Design review of the part built by this model. Coordinates are the model's own, in mm. Give positions to 0.01 mm unless a question says otherwise; leave off trailing zeros. Write each loop counter-clockwise with the first axis right and the second up, starting at its lowest first coordinate (ties: lowest second). Pieces come first, ordered by that corner, then holes. Notation, with made-up numbers: (48, 27) -> (62, 27) arc R27 ccw to (62, 56) -> close; hole circle Ø6 at (38.25, 7.25). An arc over 180 degrees is marked (long way). Answer as a JSON object with one key per item and string values.
```python
from build123d import *

# Parameters (mm, degrees)
F0_R     = 69.85
F0_R_2   = 11.1125
F1_DEPTH = 12.7
F2_SIZE  = 1.5875
F3_SIZE  = 1.5875


with BuildPart() as f1:
    # F0 (on Right) → F1 (new body)
    with BuildSketch(Plane.YZ):
        Circle(F0_R)
        Circle(F0_R_2, mode=Mode.SUBTRACT)
    extrude(amount=F1_DEPTH)

    # F2
    f2_edges = [f1.edges().sort_by_distance(p)[0] for p in [
        (0, -11.1125, 0),
        (12.7, -11.1125, 0),
    ]]
    chamfer(f2_edges, length=F2_SIZE)

    # F3
    f3_edges = [f1.edges().sort_by_distance(p)[0] for p in [
        (0, -69.85, 0),
        (12.7, -69.85, 0),
    ]]
    chamfer(f3_edges, length=F3_SIZE)


solid = f1.part
```
(1) We need section A-A, the plane z = 0. State the section outline as (x, y) points, then the cut area to 3 significant figures.
Here are the results:
{"outline": "(0, -68.26) -> (1.59, -69.85) -> (11.11, -69.85) -> (12.7, -68.26) -> (12.7, -12.7) -> (11.11, -11.11) -> (1.59, -11.11) -> (0, -12.7) -> close; (0, 12.7) -> (1.59, 11.11) -> (11.11, 11.11) -> (12.7, 12.7) -> (12.7, 68.26) -> (11.11, 69.85) -> (1.59, 69.85) -> (0, 68.26) -> close", "area": "1,480 mm²"}
(2) The part is to be moulded in two halves that separate along Z. For faces 1 (the cylindrical face through (6.28, 10.6, 3.34)), 2 (the cylindrical face through (6.283, -55.431, -42.503)), 3 (the flat face through (0, -1, -14)), say which applies: +Z half, -Z half, draft (parallel to the pull), parting line (faces both ways), or undercut.
Here are the results:
{"face 1": "undercut", "face 2": "parting line", "face 3": "draft"}
(3) Clearance check with flat-ended pins moving along their axes: pin 1 (5 mm diameter, centred on x = 3.5, z = -50, fed in from +Y); pin 2 (3 mm diameter, centred on x = 8.5, y = 51.5, fed in from -Z). State where each tip first meets the part, or that it passes through.
Here are the results:
{"pin 1": "stops at y = 51.21", "pin 2": "stops at z = -48.78"}
(4) For line 1 along Z through (x, y) = (8, 0); line 2 along Y through (x, z) = (6, -9); line 3 along Z through (x, y) = (11, -58), list the stretches that pass through material, from the lowest coordinate up.
Here are the results:
{"line 1": "z = -69.85 to -11.11, 11.11 to 69.85", "line 2": "y = -69.27 to -6.52, 6.52 to 69.27", "line 3": "z = -38.92 to 38.92"}
